Here's how the part is built. I have some questions about the finished solid (model axes, mm). A direction names the side the tool comes from. Coordinates: 2 decimals unless noted, no trailing zeros. Write each loop counter-clockwise with the first axis right and the second up, starting at its lowest first coordinate (ties: lowest second). Pieces come first, ordered by that corner, then holes.
Item 1: For faces 4 (the face through (4.1, -4.32, 6.7)), 5 (the face through (-0.6, -4.15, 2.44)), 6 (the face through (1.958, 4.02, 9.715)), 7 (the face through (-0.604, -4.133, 9.583)), 8 (the face through (1, 0, 3.7)), which set-ups out of +Z, -Z, +X, -X, +Y, -Y let a thin tool reach every point of the face, with its end or its side?
Item 2: We'd pull the mould along Y, two halves only. Please class faces 1 (the face through (3.866, 0, 6)), 2 (the face through (0.574, 0.496, 2.862)), 3 (the face through (-5.32, 0.1, 3.35)): +Y half, -Y half, draft (parallel to the pull), parting line (faces both ways), or undercut.
Item 3: If I drill on line 1 (Z direction, x = 1.75, y = -2); line 2 (Y direction, x = 16.75, z = 7.5); line 3 (Z direction, x = 15.5, y = 3.25), over which ranges is the centre line in solid material (lowest first)?
Item 4: If we section it at C-C (y = 0): Please give me the cut outline in (x, z).
Item 5: I'm going to push flat-ended pins straight in: pin 1 Ø3.5 at (x, y) = (11.5, -0.5) entering from +Z; pin 2 Ø0.6 at (x, z) = (-0.5, 3.5) entering from -Y; pin 3 Ø1.5 at (y, z) = (-3, 6) entering from -X; pin 4 Ø4 at (y, z) = (3, 7.5) entering from +X. Where does each tip first touch, or does it pass through?
Item 6: If we section it at D-D (z = 7): Please give me the cut outline in (x, y).
Item 7: If we section it at A-A (x = 1.75): Please give me the cut outline in (y, z), then the cut area to 3 significant figures.
from build123d import *

# Parameters (mm, degrees)
BOSS_EXTRUDE1_OUTLINE_W = 40
BOSS_EXTRUDE1_OUTLINE_H = 12
BOSS_EXTRUDE1_DEPTH     = 10
CUT_EXTRUDE1_DEPTH      = 6
SKETCH3_R               = 1.35
CUT_EXTRUDE2_DEPTH      = 27
SKETCH4_W               = 40.172055773
SKETCH4_H               = 12
CUT_EXTRUDE3_DEPTH      = 2
CUT_EXTRUDE6_DEPTH      = 25
CUT_EXTRUDE9_DEPTH      = 20
SKETCH14_W              = 8
SKETCH14_H              = 1.679652208
CUT_EXTRUDE10_DEPTH     = 24.151673806
BOSS_EXTRUDE4_START     = -4
BOSS_EXTRUDE4_DEPTH     = 8
FILLET7_R               = 0.5
SKETCH18_W              = 15
SKETCH18_H              = 1.5
BOSS_EXTRUDE7_DEPTH     = 8
SKETCH23_W              = 8
SKETCH23_H              = 8.64
BOSS_EXTRUDE9_DEPTH     = 5
SKETCH24_R              = 1.65
CUT_EXTRUDE13_DEPTH     = 23.313145193
SKETCH25_W              = 15.080583778
SKETCH25_H              = 4.25
CUT_EXTRUDE14_DEPTH     = 25.552672093
FILLET13_R              = 1


# Read off the part's stored shape, not the designer's step: Boss-Extrude1, Boss-Extrude4
with BuildPart() as part:
    # Boss-Extrude1 outline → Boss-Extrude1 (new body)
    with BuildSketch(Plane.XY):
        Rectangle(BOSS_EXTRUDE1_OUTLINE_W, BOSS_EXTRUDE1_OUTLINE_H)
    extrude(amount=BOSS_EXTRUDE1_DEPTH)

    # Sketch2 → Cut-Extrude1 (cut)
    with BuildSketch(Plane.XY.offset(10)):
        with BuildLine():
            Line((20.002042678, 3.45), (20, -3.45))
            Line((20, -3.45), (9.967611838, -3.45))
            ThreePointArc((9.967611838, -3.45), (6.517611838, 0), (9.967611838, 3.45))
            Line((9.967611838, 3.45), (20.002042678, 3.45))
        make_face()
    extrude(amount=-CUT_EXTRUDE1_DEPTH, mode=Mode.SUBTRACT)

    # Sketch3 → Cut-Extrude2 (cut)
    with BuildSketch(Plane.XY.offset(4)):
        with Locations((13.967611838, 0)):
            Circle(SKETCH3_R)
        with Locations((9.967611838, 0)):
            Circle(SKETCH3_R)
    extrude(amount=-CUT_EXTRUDE2_DEPTH, mode=Mode.SUBTRACT)

    # Sketch4 → Cut-Extrude3 (cut)
    with BuildSketch(Plane(origin=(0, 0, 0), x_dir=(-1, 0, 0), z_dir=(0, 0, -1))):
        with Locations((0.086027887, 0)):
            Rectangle(SKETCH4_W, SKETCH4_H)
    extrude(amount=-CUT_EXTRUDE3_DEPTH, mode=Mode.SUBTRACT)

    # Sketch7 → Cut-Extrude6 (cut)
    with BuildSketch(Plane.ZY.offset(20)):
        Polygon((2, 6), (2, 2.309401077), (2, -2.309401077), (2, -6), (10, -6), (10, -2.309401077), (10, 2.309401077), (10, 6), align=None)
        Polygon((9.256150484, -1.879939359), (6, -3.759878717), (2.743849516, -1.879939359), (2.743849516, 1.879939359), (6, 3.759878717), (9.256150484, 1.879939359), align=None, mode=Mode.SUBTRACT)
    extrude(amount=-CUT_EXTRUDE6_DEPTH, mode=Mode.SUBTRACT)

    # Sketch11 → Cut-Extrude9 (cut)
    with BuildSketch(Plane.ZY.offset(20)):
        Polygon((10, -2.309401077), (10, 2.309401077), (6, 4.618802154), (2, 2.309401077), (2, -2.309401077), (6, -4.618802154), align=None)
    extrude(amount=-CUT_EXTRUDE9_DEPTH, mode=Mode.SUBTRACT)

    # Sketch14 → Cut-Extrude10 (cut, through all)
    with BuildSketch(Plane.ZY):
        with Locations((6, -5.160173896)):
            Rectangle(SKETCH14_W, SKETCH14_H)
    cut_extrude10 = extrude(amount=-CUT_EXTRUDE10_DEPTH, mode=Mode.SUBTRACT)

    # Mirror4: Cut-Extrude10 across plane
    add(cut_extrude10.mirror(Plane.ZX), mode=Mode.SUBTRACT)

    # Boss-Extrude4 outline → Boss-Extrude4 (add)
    with BuildSketch(Plane.XY.offset(6).offset(BOSS_EXTRUDE4_START)):
        with BuildLine():
            ThreePointArc((-1, 4.320347792), (-5.320347792, 0), (-1, -4.320347792))
            Line((-1, -4.320347792), (0, -4.320347792))
            Line((0, -4.320347792), (0, -4.203023322))
            ThreePointArc((0, -4.203023322), (3.320347792, 0), (0, 4.203023322))
            Line((0, 4.203023322), (0, 4.320347792))
            Line((0, 4.320347792), (-1, 4.320347792))
        make_face()
    extrude(amount=BOSS_EXTRUDE4_DEPTH)

    # Fillet7
    fillet7_edges = [part.edges().sort_by_distance(p)[0] for p in [
        (3.06403913, 3.759878717, 6),
        (3.944944283, 1.879939359, 2.743849516),
        (3.944944283, -1.879939359, 2.743849516),
        (3.06403913, -3.759878717, 6),
        (3.944944283, -1.879939359, 9.256150484),
        (3.944944283, 1.879939359, 9.256150484),
    ]]
    fillet(fillet7_edges, radius=FILLET7_R)

    # Sketch18 → Boss-Extrude7 (add)
    with BuildSketch(Plane.XY.offset(10)):
        with Locations((12.5, 5.070347792)):
            Rectangle(SKETCH18_W, SKETCH18_H)
        with Locations((12.5, -5.070347792)):
            Rectangle(SKETCH18_W, SKETCH18_H)
    extrude(amount=-BOSS_EXTRUDE7_DEPTH)

    # Sketch23 → Boss-Extrude9 (add)
    with BuildSketch(Plane(origin=(0, 0, 0), x_dir=(0, 0, -1), z_dir=(1, 0, 0))):
        with Locations((-6, 0.000347792)):
            Rectangle(SKETCH23_W, SKETCH23_H)
    extrude(amount=BOSS_EXTRUDE9_DEPTH)

    # Sketch24 → Cut-Extrude13 (cut, through all)
    with BuildSketch(Plane.XY.offset(10)):
        with Locations((-1, 0)):
            Circle(SKETCH24_R)
    extrude(amount=-CUT_EXTRUDE13_DEPTH, mode=Mode.SUBTRACT)

    # Sketch25 → Cut-Extrude14 (cut, through all)
    with BuildSketch(Plane(origin=(0, 4.320347792, 0), x_dir=(1, 0, 0), z_dir=(0, 1, 0))):
        with Locations((-3.674163861, -5.825)):
            Rectangle(SKETCH25_W, SKETCH25_H)
    extrude(amount=-CUT_EXTRUDE14_DEPTH, mode=Mode.SUBTRACT)

    # Fillet13
    fillet13_edges = [part.edges().sort_by_distance(p)[0] for p in [
        (-5.320347792, 0, 2),
        (2.5, 4.320347792, 10),
        (-0.5, -4.320347792, 2),
        (2.5, 4.320347792, 2),
        (-5.320347792, 0, 10),
        (-0.5, -4.320347792, 10),
        (12.5, 5.820347792, 2),
        (5, 5.820347792, 6),
        (12.5, 5.820347792, 10),
        (5, -5.820347792, 6),
        (12.5, -5.820347792, 2),
        (12.5, -5.820347792, 10),
        (0, -4.32, 2),
        (0, -4.32, 10),
        (2.5, -4.319652208, 10),
        (2.5, -4.319652208, 2),
    ]]
    fillet(fillet13_edges, radius=FILLET13_R)


solid = part.part
Answer list:
1. face 4: +Z, -Z, -X, -Y
1. face 5: -Z, -X, -Y
1. face 6: +Z, -X, +Y
1. face 7: +Z, -X, -Y
1. face 8: -X, +Y, -Y
2. face 1: draft
2. face 2: undercut
2. face 3: parting line
3. line 1: z = 2 to 3.7, 7.95 to 10
3. line 2: y = -5.82 to -3.45, 3.45 to 5.82
3. line 3: z = 2 to 4
4. outline: (-5.32, 3) arc R1 ccw to (-4.32, 2) - (-2.65, 2) - (-2.65, 3.7) - (-5.32, 3.7) - close; (-5.32, 7.95) - (-2.65, 7.95) - (-2.65, 10) - (-4.32, 10) arc R1 ccw to (-5.32, 9) - close; (0.65, 2) - (8.62, 2) - (8.62, 4) - (6.52, 4) - (6.52, 10) - (0.65, 10) - (0.65, 7.95) - (3.87, 7.95) - (3.87, 3.7) - (0.65, 3.7) - close; (11.32, 2) - (12.62, 2) - (12.62, 4) - (11.32, 4) - close; (15.32, 2) - (20, 2) - (20, 4) - (15.32, 4) - close
5. pin 1: stops at z = 4
5. pin 2: stops at y = -4.32
5. pin 3: stops at x = 3.87
5. pin 4: stops at x = 20
6. outline: (3.87, -4.32) - (5, -4.32) - (5, -4.82) arc R1 ccw to (6, -5.82) - (20, -5.82) - (20, -3.45) - (9.97, -3.45) arc R3.45 cw to (9.97, 3.45) - (20, 3.45) - (20, 5.82) - (6, 5.82) arc R1 ccw to (5, 4.82) - (5, 4.32) - (3.87, 4.32) - close
7. outline: (-4.32, 3) arc R1 ccw to (-3.32, 2) - (3.32, 2) arc R1 ccw to (4.32, 3) - (4.32, 3.7) - (-4.32, 3.7) - close; (-4.32, 7.95) - (4.32, 7.95) - (4.32, 9) arc R1 ccw to (3.32, 10) - (-3.32, 10) arc R1 ccw to (-4.32, 9) - close
7. area: 31.5 mm2
